The model under review builds one solid part; all positions refer to its coordinate system, in mm. A direction names the side the tool comes from. Give positions to 0.01 mm unless a question says otherwise; leave off trailing zeros. Order: outer loops, then holes, each group sorted by start corner. A loop starts at its lowest first (then second) coordinate and runs counter-clockwise, first axis right, second up.
```python
from build123d import *

# Parameters (mm, degrees)
SKETCH_1_W           = 42
SKETCH_1_H           = 42
EXTRUDE_1_DEPTH      = 48
CUT_EXTRUDE_START    = 48
CUT_EXTRUDE_1_DEPTH  = 48
CUT_EXTRUDE_START_2  = 9.5
CUT_EXTRUDE_2_DEPTH  = 31
CUT_EXTRUDE_START_3  = -21
SKETCH_4_W           = 33
SKETCH_4_H           = 31
CUT_EXTRUDE_3_DEPTH  = 0.1
CUT_EXTRUDE_START_4  = 21
SKETCH_5_W           = 33
SKETCH_5_H           = 31
CUT_EXTRUDE_4_DEPTH  = 0.1
SKETCH_6_W           = 33
SKETCH_6_H           = 31
CUT_EXTRUDE_5_DEPTH  = 0.1
SKETCH_7_W           = 33
SKETCH_7_H           = 31
CUT_EXTRUDE_6_DEPTH  = 0.1
SKETCH_17_R          = 4.75
CUT_EXTRUDE_9_DEPTH  = 3
EXTRUDE_START        = 48
SKETCH_18_R          = 11
EXTRUDE_2_DEPTH      = 2
CUT_EXTRUDE_START_5  = 50
SKETCH_20_R          = 2.5
CUT_EXTRUDE_10_DEPTH = 47
EXTRUDE_START_2      = 21
SKETCH_21_W          = 15.3
SKETCH_21_H          = 2.2
EXTRUDE_3_DEPTH      = 4
SKETCH_22_W          = 15.3
SKETCH_22_H          = 5.5
EXTRUDE_4_DEPTH      = 4
CUT_EXTRUDE_11_DEPTH = 4
EXTRUDE_START_3      = -7.65
EXTRUDE_5_DEPTH      = 15.3
SKETCH_8_R           = 1.5
CUT_EXTRUDE_12_DEPTH = 108.715994507


with BuildPart() as part:
    # 草图1 → 凸台-拉伸1 (new body)
    with BuildSketch(Plane(origin=(0, 0, 0), x_dir=(1, 0, 0), z_dir=(0, 1, 0))):
        Rectangle(SKETCH_1_W, SKETCH_1_H)
    extrude(amount=EXTRUDE_1_DEPTH)

    # 草图2 → 切除-拉伸1 (cut)
    with BuildSketch(Plane(origin=(0, 0, 0), x_dir=(1, 0, 0), z_dir=(0, 1, 0)).offset(CUT_EXTRUDE_START)):
        Polygon((-21, 21), (-16.5, 21), (-21, 16.5), align=None)
        Polygon((21, 16.5), (21, 21), (16.5, 21), align=None)
        Polygon((21, -21), (16.5, -21), (21, -16.5), align=None)
        Polygon((-21, -16.5), (-21, -21), (-16.5, -21), align=None)
    extrude(amount=-CUT_EXTRUDE_1_DEPTH, mode=Mode.SUBTRACT)

    # 草图3 → 切除-拉伸2 (cut)
    with BuildSketch(Plane(origin=(0, 0, 0), x_dir=(1, 0, 0), z_dir=(0, 1, 0)).offset(CUT_EXTRUDE_START_2)):
        Polygon((-21, 13.5), (-21, 21), (-13.5, 21), align=None)
        Polygon((13.5, 21), (21, 13.5), (21, 21), align=None)
        Polygon((21, -13.5), (21, -21), (13.5, -21), align=None)
        Polygon((-13.5, -21), (-21, -13.5), (-21, -21), align=None)
    extrude(amount=CUT_EXTRUDE_2_DEPTH, mode=Mode.SUBTRACT)

    # 草图4 → 切除-拉伸3 (cut)
    with BuildSketch(Plane.XY.offset(CUT_EXTRUDE_START_3)):
        with Locations((0, 25)):
            Rectangle(SKETCH_4_W, SKETCH_4_H)
    extrude(amount=CUT_EXTRUDE_3_DEPTH, mode=Mode.SUBTRACT)

    # 草图5 → 切除-拉伸4 (cut)
    with BuildSketch(Plane.XY.offset(CUT_EXTRUDE_START_4)):
        with Locations((0, 25)):
            Rectangle(SKETCH_5_W, SKETCH_5_H)
    extrude(amount=-CUT_EXTRUDE_4_DEPTH, mode=Mode.SUBTRACT)

    # 草图6 → 切除-拉伸5 (cut)
    with BuildSketch(Plane(origin=(0, 0, 0), x_dir=(0, 0, -1), z_dir=(1, 0, 0)).offset(CUT_EXTRUDE_START_3)):
        with Locations((0, 25)):
            Rectangle(SKETCH_6_W, SKETCH_6_H)
    extrude(amount=CUT_EXTRUDE_5_DEPTH, mode=Mode.SUBTRACT)

    # 草图7 → 切除-拉伸6 (cut)
    with BuildSketch(Plane(origin=(0, 0, 0), x_dir=(0, 0, -1), z_dir=(1, 0, 0)).offset(CUT_EXTRUDE_START_4)):
        with Locations((0, 25)):
            Rectangle(SKETCH_7_W, SKETCH_7_H)
    extrude(amount=-CUT_EXTRUDE_6_DEPTH, mode=Mode.SUBTRACT)

    # 草图17 → 切除-拉伸9 (cut)
    with BuildSketch(Plane(origin=(0, 0, 0), x_dir=(1, 0, 0), z_dir=(0, 1, 0))):
        with Locations(Location((0, 0, 0), (0, 0, 270))):
            Circle(SKETCH_17_R)
    extrude(amount=CUT_EXTRUDE_9_DEPTH, mode=Mode.SUBTRACT)

    # 草图18 → 凸台-拉伸2 (add)
    with BuildSketch(Plane(origin=(0, 0, 0), x_dir=(1, 0, 0), z_dir=(0, 1, 0)).offset(EXTRUDE_START)):
        with Locations(Location((0, 0, 0), (0, 0, 90))):
            Circle(SKETCH_18_R)
    extrude(amount=EXTRUDE_2_DEPTH)

    # 草图20 → 切除-拉伸10 (cut)
    with BuildSketch(Plane(origin=(0, 0, 0), x_dir=(1, 0, 0), z_dir=(0, 1, 0)).offset(CUT_EXTRUDE_START_5)):
        with Locations(Location((0, 0, 0), (0, 0, 270))):
            Circle(SKETCH_20_R)
    extrude(amount=-CUT_EXTRUDE_10_DEPTH, mode=Mode.SUBTRACT)

    # 草图21 → 凸台-拉伸3 (add)
    with BuildSketch(Plane.XY.offset(EXTRUDE_START_2)):
        with Locations((0, 1.1)):
            Rectangle(SKETCH_21_W, SKETCH_21_H)
    extrude(amount=EXTRUDE_3_DEPTH)

    # 草图22 → 凸台-拉伸4 (add)
    with BuildSketch(Plane.XY.offset(EXTRUDE_START_2)):
        with Locations((0, 6.75)):
            Rectangle(SKETCH_22_W, SKETCH_22_H)
    extrude(amount=EXTRUDE_4_DEPTH)

    # 草图23 → 切除-拉伸11 (cut)
    with BuildSketch(Plane.XY.offset(CUT_EXTRUDE_START_4)):
        Polygon((-6.65, 8.5), (-6.65, 5), (6.65, 5), (6.65, 8.5), (4, 8.5), (4, 9.5), (-4, 9.5), (-4, 8.5), align=None)
    extrude(amount=CUT_EXTRUDE_11_DEPTH, mode=Mode.SUBTRACT)

    # 草图26 → 凸台-拉伸5 (add)
    with BuildSketch(Plane(origin=(0, 0, 0), x_dir=(0, 0, -1), z_dir=(1, 0, 0)).offset(EXTRUDE_START_3)):
        Polygon((-21, 9.5), (-20.9, 9.5), (-20.9, 9.601292788), align=None)
    extrude(amount=EXTRUDE_5_DEPTH)

    # 草图8 → 切除-拉伸12 (cut, through all)
    with BuildSketch(Plane(origin=(0, 0, 0), x_dir=(1, 0, 0), z_dir=(0, 1, 0)).offset(CUT_EXTRUDE_START)):
        with Locations(Location((-15.5, 15.5, 0), (0, 0, 90))):
            Circle(SKETCH_8_R)
        with Locations(Location((15.5, 15.5, 0), (0, 0, 90))):
            Circle(SKETCH_8_R)
        with Locations(Location((-15.5, -15.5, 0), (0, 0, 90))):
            Circle(SKETCH_8_R)
        with Locations(Location((15.5, -15.5, 0), (0, 0, 90))):
            Circle(SKETCH_8_R)
    extrude(amount=-CUT_EXTRUDE_12_DEPTH, mode=Mode.SUBTRACT)


solid = part.part
```
1. For faces 4 (the flat face through (0, 2.2, 23)), 5 (the flat face through (5, 8.5, 23)), 6 (the flat face through (-19, 40.5, 17)), 7 (the flat face through (17.2, 24.8, -17.3)), list the 3-axis set-ups (+Z, -Z, +X, -X, +Y, -Y) from which the entire face can be reached by the end or side of a thin tool; tool diameter is ignored.
2. Take a section at B-B (z = 15.5). Write out the cut boundary in (x, y).
3. Draft analysis for pull direction Y (two halves, no side actions). For faces 1 (the flat face through (-18.7, 44.3, -18.8)), 2 (the flat face through (0, 7, 21)), 3 (the flat face through (-2, 3, 2)), state which applies: pulls with the +Y half, pulls with the -Y half, needs draft (parallel to the pull), parting line crosses it, or undercut.
4. Insertion check: pin 1 (4.5 mm diameter, centred on x = -3, z = 23.5, fed in from +Y); pin 2 (10 mm diameter, centred on x = 16, z = -14.5, fed in from +Y); pin 3 (4 mm diameter, centred on x = -1, y = 25.5, fed in from -Z). Each pin has a flat end and moves straight along its axis. Give the tip position at first contact, or say it passes through.
5. Take a section at D-D (y = 31.5). Write out the cut boundary in (x, z).
6. Take a section at C-C (x = -15.5). Write out the cut boundary in (y, z).
7. To check wall thickness, follow line 1 (X direction, y = 37, z = 15.5); line 2 (Z direction, x = 15, y = 31). State the ranges of each line that lie inside material, in increasing order.
Answer:
1. face 4: +Z, +X, -X
1. face 5: +Z
1. face 6: none
1. face 7: -Z, +X
2. outline: (-21, 0) - (-17, 0) - (-17, 48) - (-21, 48) - (-21, 40.5) - (-19, 40.5) - (-19, 9.5) - (-21, 9.5) - close; (-14, 0) - (14, 0) - (14, 48) - (-14, 48) - close; (17, 0) - (21, 0) - (21, 9.5) - (19, 9.5) - (19, 40.5) - (21, 40.5) - (21, 48) - (17, 48) - close
3. face 1: needs draft
3. face 2: undercut
3. face 3: pulls with the -Y half
4. pin 1: stops at y = 9.5
4. pin 2: stops at y = 48
4. pin 3: stops at z = -20.9
5. outline: (-20.9, -13.6) - (-13.6, -20.9) - (13.6, -20.9) - (20.9, -13.6) - (20.9, 13.6) - (13.6, 20.9) - (-13.6, 20.9) - (-20.9, 13.6) - close; hole circle Ø3 at (-15.5, -15.5); hole circle Ø3 at (-15.5, 15.5); hole circle Ø5 at (0, 0); hole circle Ø3 at (15.5, -15.5); hole circle Ø3 at (15.5, 15.5)
6. outline: (0, -21) - (9.5, -21) - (9.5, -19) - (40.5, -19) - (40.5, -21) - (48, -21) - (48, -17) - (0, -17) - close; (0, -14) - (48, -14) - (48, 14) - (0, 14) - close; (0, 17) - (48, 17) - (48, 21) - (40.5, 21) - (40.5, 19) - (9.5, 19) - (9.5, 21) - (0, 21) - close
7. line 1: x = -19 to -17, -14 to 14, 17 to 19
7. line 2: z = -19.5 to -16.91, -14.09 to 14.09, 16.91 to 19.5
